Check sheet for the drawn part. Datum: minimum x, y, z corner. Units: mm. Give positions to 0.01 mm unless a question says otherwise; leave off trailing zeros. Order: outer loops, then holes, each group sorted by start corner. A loop starts at its lowest first (then second) coordinate and runs counter-clockwise, first axis right, second up. Notation, with made-up numbers: (-15, 45) - (31, 45) arc R25 ccw to (31, 66) - close; hole circle Ø5 at (89, 76). An arc over 180 degrees is marked (long way). Answer as a JSON object with one key per item and string values. Group by question number.
(1) Section check D-D (x = 10). Record the boundary of the cut face in (y, z).
(2) Thickness scan on line 1 (Y direction, x = 10, z = 1.3); line 2 (X direction, y = 29.5, z = 3.55); line 3 (Y direction, x = 22, z = 3.1). Record the ranges inside material, lowest first.
(3) Section check A-A (y = 20). Record the boundary of the cut face in (x, z).
(4) Depth check by flat-ended pin: pin 1 Ø1.5 at (x, y) = (29.5, 10.5) entering from +Z; pin 2 Ø4 at (x, y) = (30, 10) entering from +Z; pin 3 Ø1 at (y, z) = (13.5, 1.5) entering from -X. Enter the tip coordinate at first touch or a pass-through.
(5) Section check C-C (z = 1.3). Record the boundary of the cut face in (x, y).
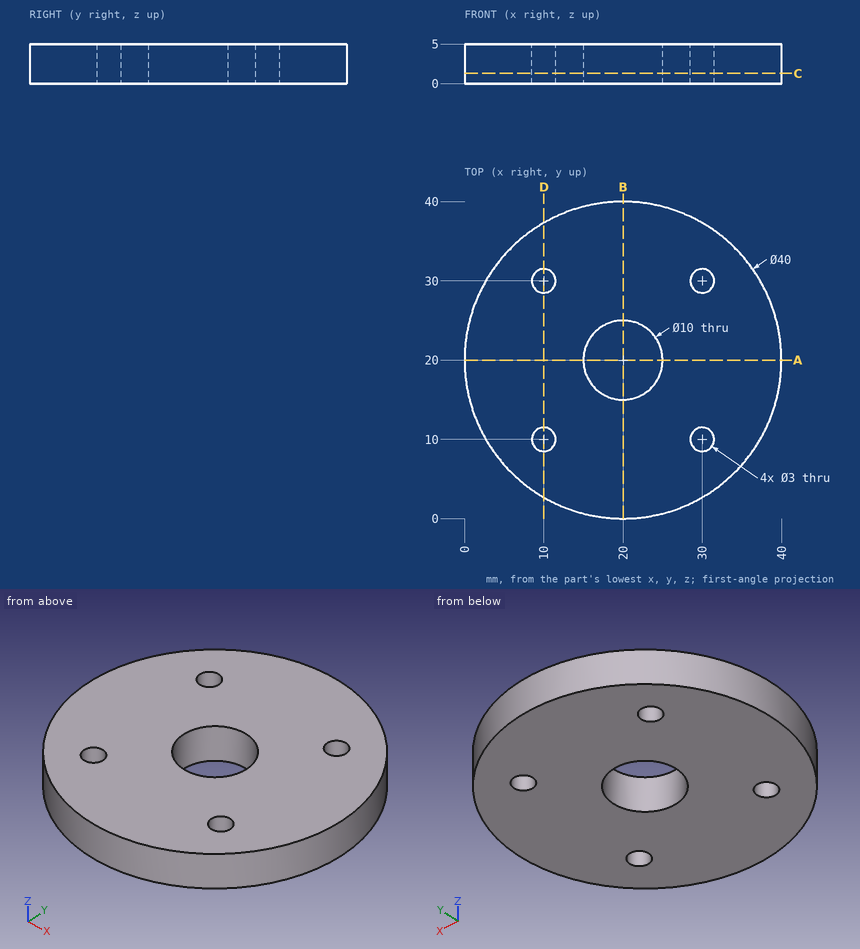
Solutions:
{
 "1": {"outline": "(2.68, 0) - (8.5, 0) - (8.5, 5) - (2.68, 5) - close; (11.5, 0) - (28.5, 0) - (28.5, 5) - (11.5, 5) - close; (31.5, 0) - (37.32, 0) - (37.32, 5) - (31.5, 5) - close"},
 "2": {"line 1": "y = 2.68 to 8.5, 11.5 to 28.5, 31.5 to 37.32", "line 2": "x = 2.4 to 8.59, 11.41 to 28.59, 31.41 to 37.6", "line 3": "y = 0.1 to 15.42, 24.58 to 39.9"},
 "3": {"outline": "(0, 0) - (15, 0) - (15, 5) - (0, 5) - close; (25, 0) - (40, 0) - (40, 5) - (25, 5) - close"},
 "4": {"pin 1": "passes through", "pin 2": "stops at z = 5", "pin 3": "stops at x = 0.92"},
 "5": {"outline": "circle Ø40 at (20, 20); hole circle Ø3 at (10, 10); hole circle Ø3 at (10, 30); hole circle Ø10 at (20, 20); hole circle Ø3 at (30, 10); hole circle Ø3 at (30, 30)"}
}
